```python
from build123d import *

# Parameters (mm, degrees)
SKETCH1_W           = 99.30160125
SKETCH1_H           = 60.173202502
SKETCH1_R           = 2.413
BOSS_EXTRUDE1_DEPTH = 2.54
SKETCH1_3_R         = 2.413
CUT_EXTRUDE1_DEPTH  = 2.54
SKETCH1_4_R         = 4.056034091
CUT_EXTRUDE2_DEPTH  = 2.032
FILLET1_R           = 2.54


with BuildPart() as part:
    # Sketch1 → Boss-Extrude1 (new body)
    with BuildSketch(Plane.XY):
        with Locations((2.344221604, 0)):
            Rectangle(SKETCH1_W, SKETCH1_H)
        with Locations((46.794221604, -24.885800625)):
            Circle(SKETCH1_R, mode=Mode.SUBTRACT)
    extrude(amount=BOSS_EXTRUDE1_DEPTH)

    # Sketch1_3 → Cut-Extrude1 (cut)
    with BuildSketch(Plane.XY):
        with Locations((-42.105778396, 24.885800625)):
            Circle(SKETCH1_3_R)
        with Locations((46.794221604, 24.885800625)):
            Circle(SKETCH1_3_R)
    extrude(amount=CUT_EXTRUDE1_DEPTH, mode=Mode.SUBTRACT)

    # Sketch1_4 → Cut-Extrude2 (cut)
    with BuildSketch(Plane.XY):
        with Locations((-42.105778396, 24.885800625)):
            Circle(SKETCH1_4_R)
        with Locations((46.794221604, 24.885800625)):
            Circle(SKETCH1_4_R)
        with Locations((46.794221604, -24.885800625)):
            Circle(SKETCH1_4_R)
    extrude(amount=CUT_EXTRUDE2_DEPTH, mode=Mode.SUBTRACT)

    # Fillet1
    fillet1_edges = [part.edges().sort_by_distance(p)[0] for p in [
        (-47.306579021, 30.086601251, 1.27),
        (51.995022229, 30.086601251, 1.27),
        (51.995022229, -30.086601251, 1.27),
        (-47.306579021, -30.086601251, 1.27),
    ]]
    fillet(fillet1_edges, radius=FILLET1_R)


solid = part.part
```
Geometry check sheet. Reference: the model listing, model coordinates, mm. A direction names the side the tool comes from. Coordinates: 2 decimals unless noted, no trailing zeros. Loops run counter-clockwise (first coordinate to the right, second up) from the corner with the lowest first, then second, coordinate; pieces in that order, holes last. Notation, with made-up numbers: (59.25, 69.25) -> (79.25, 69.25) arc R38 ccw to (79.25, 108.25) -> close; hole circle Ø5 at (42, 47.25). An arc over 180 degrees is marked (long way). Put each result on its own line as item: value.
1) Cross-section at B-B on z = 0.7. Record the boundary of the cut face in (x, y).
Result set:
outline: (-47.31, -27.55) arc R2.54 ccw to (-44.77, -30.09) -> (49.46, -30.09) arc R2.54 ccw to (52, -27.55) -> (52, 27.55) arc R2.54 ccw to (49.46, 30.09) -> (-44.77, 30.09) arc R2.54 ccw to (-47.31, 27.55) -> close; hole circle Ø8.11 at (-42.11, 24.89); hole circle Ø8.11 at (46.79, -24.89); hole circle Ø8.11 at (46.79, 24.89)
2) Tool access check on faces 1 (the flat face through (2, 30.087, 1)), 2 (the flat face through (-40, 23, 2.032)). Record the directions out of +Z, -Z, +X, -X, +Y, -Y that give a thin tool (end or side, any length) a straight path to the whole face; none if there is none.
Result set:
face 1: +Z, -Z, +X, -X, +Y
face 2: -Z
3) Release check for a two-part mould opening along Y. For faces 3 (the cylindrical face through (-39.93, 28.31, 1)), 4 (the cylindrical face through (51.231, 29.362, 1.288)), 5 (the flat face through (2, -30.087, 1)) record: released by +Y, released by -Y, zero draft, split by the parting line, or undercut.
Result set:
face 3: undercut
face 4: released by +Y
face 5: released by -Y
4) Thickness scan on line 1 (X direction, y = 26, z = 1.15); line 2 (Z direction, x = 44, y = 27.5). Record the ranges inside material, lowest first.
Result set:
line 1: x = -47.31 to -46.01, -38.21 to 42.89, 50.69 to 52
line 2: z = 2.03 to 2.54
5) Cross-section at A-A on y = 26. Record the boundary of the cut face in (x, z).
Result set:
outline: (-47.31, 0) -> (-46.01, 0) -> (-46.01, 2.03) -> (-44.25, 2.03) -> (-44.25, 2.54) -> (-47.31, 2.54) -> close; (-39.97, 2.03) -> (-38.21, 2.03) -> (-38.21, 0) -> (42.89, 0) -> (42.89, 2.03) -> (44.65, 2.03) -> (44.65, 2.54) -> (-39.97, 2.54) -> close; (48.93, 2.03) -> (50.69, 2.03) -> (50.69, 0) -> (52, 0) -> (52, 2.54) -> (48.93, 2.54) -> close
6) Gauge pin test, flat ends, axial feed: pin 1 Ø13 at (x, y) = (46.79, 24.89) entering from -Z; pin 2 Ø4 at (x, y) = (47.5, -24.5) entering from -Z. Record the tip position at first contact, or that the pin passes through.
Result set:
pin 1: stops at z = 0
pin 2: stops at z = 2.03
